Geometry: see drawing. Coordinates: mm, zero at the bounding-box minimum. Give positions to 0.01 mm unless a question says otherwise; leave off trailing zeros. Write each loop counter-clockwise with the first axis right and the second up, starting at its lowest first coordinate (ties: lowest second). Pieces come first, ordered by that corner, then holes. Notation, with made-up numbers: (-31.75, 37) -> (-21.75, 37) arc R10 ccw to (-21.75, 56) -> close; hole circle Ø9 at (77, 88). An arc over 180 degrees is marked (long way). Answer as a JSON object with one key per item and string values. Group by question number.
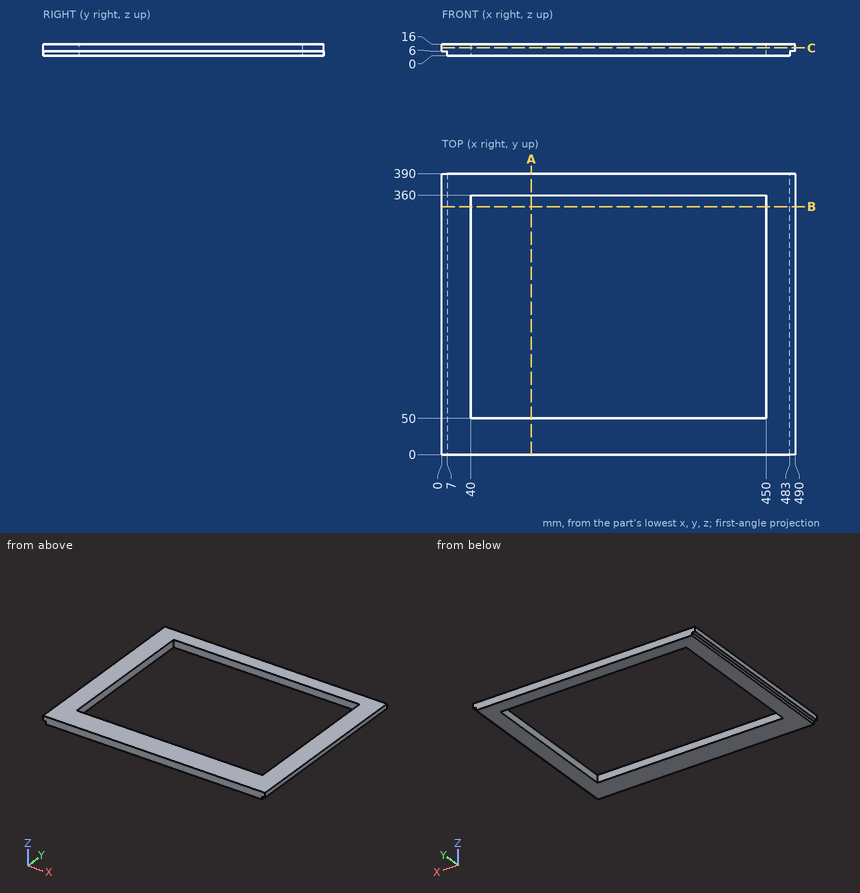
1. Contact query for flat-ended pins moving along their axis: pin 1 Ø1.8 at (y, z) = (262, 4) entering from -X; pin 2 Ø5 at (y, z) = (261, 3) entering from +X; pin 3 Ø2 at (x, y) = (487, 97.5) entering from -Z. Output: stop coordinate, or through.
2. Section B-B (y = 344). Return the cut outline in (x, z).
3. Section A-A (x = 124). Return the cut outline in (y, z).
4. Line query: line 1 (Y direction, x = 133, z = 8.5); line 2 (X direction, y = 255, z = 7.5); line 3 (X direction, y = 331.5, z = 2). Output: solid intervals per line, ascending.
5. Section C-C (z = 10.5). Return the cut outline in (x, y), plus the area to 3 significant figures.
Working result:
{
 "1": {"pin 1": "stops at x = 7", "pin 2": "stops at x = 483", "pin 3": "stops at z = 6"},
 "2": {"outline": "(0, 6) -> (7, 6) -> (7, 0) -> (40, 0) -> (40, 16) -> (0, 16) -> close; (450, 0) -> (483, 0) -> (483, 6) -> (490, 6) -> (490, 16) -> (450, 16) -> close"},
 "3": {"outline": "(0, 0) -> (50, 0) -> (50, 16) -> (0, 16) -> close; (360, 0) -> (390, 0) -> (390, 16) -> (360, 16) -> close"},
 "4": {"line 1": "y = 0 to 50, 360 to 390", "line 2": "x = 0 to 40, 450 to 490", "line 3": "x = 7 to 40, 450 to 483"},
 "5": {"outline": "(0, 0) -> (490, 0) -> (490, 390) -> (0, 390) -> close; hole (40, 50) -> (450, 50) -> (450, 360) -> (40, 360) -> close", "area": "64,000 mm^2"}
}
